Autodesk Inventor part; units mm, degrees
ref_plane "YZ Plane" through (0, 0, 0) normal (1, 0, 0) x (0, 1, 0)
ref_plane "XZ Plane" through (0, 0, 0) normal (0, 1, 0) x (-1, 0, 0)
ref_plane "XY Plane" through (0, 0, 0) normal (0, 0, 1) x (1, 0, 0)
sketch "Szkic1" plane through (0, 0, 0) normal (0, 1, 0) x (-1, 0, 0)
  line L0 (0, 0) -> (12.2, 0)
  line L1 (12.2, 0) -> (12.2, -22.6)
  line L2 (12.2, -22.6) -> (0, -22.6)
  line L3 (0, -22.6) -> (0, 0)
  dimension "d0" = 12.2
  dimension "d1" = 22.6
extrude "Wyciągnięcie proste1" add sketch "Szkic1" along normal blind 22.6
sketch "Szkic2" plane through (-12.2, 0, 0) normal (0, 0, 1) x (1, 0, 0)
  line L0 (0, 22.6) -> (12.2, 22.6) construction
  line L1 (0, 22.6) -> (0, 18.5) construction
  line L2 (0, 0) -> (0, 22.6) construction
  line L3 (0, 18.5) -> (12.2, 18.5) construction
  line L4 (12.2, 0) -> (12.2, 22.6) construction
  line L5 (0, 18.5) -> (0, 16.1) construction
  line L6 (0, 18.5) -> (12.2, 18.5)
  line L7 (12.2, 18.5) -> (12.2, 16.1)
  line L8 (12.2, 16.1) -> (0, 16.1)
  line L9 (0, 16.1) -> (0, 18.5)
  dimension "d4" = 4.1
  dimension "d5" = 2.4
extrude "Wyciągnięcie proste2" add sketch "Szkic2" along normal blind 4.5
sketch "Szkic3" plane through (0, 0, -22.6) normal (0, 0, -1) x (-1, 0, 0)
  line L0 (12.2, 18.5) -> (0, 18.5)
  line L1 (0, 16.1) -> (12.2, 16.1)
  line L2 (12.2, 0) -> (12.2, 22.6)
  line L3 (0, 0) -> (0, 22.6)
  line L4 (12.2, 18.5) -> (0, 18.5)
  line L5 (0, 18.5) -> (0, 16.1)
  line L6 (0, 16.1) -> (12.2, 16.1)
  line L7 (12.2, 16.1) -> (12.2, 18.5)
extrude "Wyciągnięcie proste3" add sketch "Szkic3" along normal blind 4.5
sketch "Szkic4" plane through (-12.2, 18.5, 0) normal (0, 1, 0) x (1, 0, 0)
  line L0 (0, -4.5) -> (12.2, -4.5) construction
  line L1 (6.1, -4.5) -> (6.1, 27) construction
  line L2 (6.1, -4.5) -> (5.6, -4.5) construction
  line L3 (6.1, -4.5) -> (6.1, -2.4) construction
  circle A0 centre (6.1, -2.4) radius 1 construction
  line L4 (5.6, -4.5) -> (6.6, -4.5) construction
  line L5 (6.6, -4.5) -> (6.6, -3) construction
  line L6 (6.6, -3) -> (5.6, -3) construction
  line L7 (5.6, -3) -> (5.6, -4.5) construction
  line L8 (5.6, -4.5) -> (5.6, -3.266)
  line L9 (5.6, -4.5) -> (6.6, -4.5)
  line L10 (6.6, -4.5) -> (6.6, -3.266)
  arc A1 (6.6, -3.266) -> (5.6, -3.266) centre (6.1, -2.4) ccw
  line L11 (0, 22.6) -> (0, 0) construction
  line L12 (0, 11.3) -> (12.2, 11.3) construction
  line L13 (12.2, 0) -> (12.2, 22.6) construction
  circle A2 centre (6.1, 25) radius 1 construction
  line L14 (5.6, 27.1) -> (6.6, 27.1) construction
  line L15 (5.6, 27.1) -> (5.6, 25.866)
  line L16 (6.6, 27.1) -> (6.6, 25.866)
  line L17 (5.6, 27.1) -> (6.6, 27.1)
  line L18 (0, 27.1) -> (12.2, 27.1)
  arc A3 (5.6, 25.866) -> (6.6, 25.866) centre (6.1, 25) ccw
  dimension "d10" = 0.5
  dimension "d11" = 2.1
  dimension "d12" = 2
  dimension "d13" = 1
extrude "Wyciągnięcie proste4" cut sketch "Szkic4" against normal blind 2.4
sketch "Szkic5" plane through (0, 22.6, 0) normal (0, 1, 0) x (1, 0, 0)
  line L0 (-12.2, 0) -> (0, 0) construction
  line L1 (-6.1, 0) -> (-6.1, 6.1) construction
  circle A0 centre (-6.1, 6.1) radius 6.1 construction
  line L2 (-6.1, 0) -> (-6.1, 14.5) construction
  circle A1 centre (-6.1, 12.2) radius 2.3 construction
  arc A2 (-8.3588, 11.7664) -> (-3.8412, 11.7664) centre (-6.1, 6.1) ccw
  arc A3 (-3.8412, 11.7664) -> (-8.3588, 11.7664) centre (-6.1, 12.2) ccw
  dimension "d16" = 6.1
  dimension "d17" = 12.2
  dimension "d18" = 14.5
extrude "Wyciągnięcie proste5" add sketch "Szkic5" along normal blind 4.1
sketch "Szkic6" plane through (0, 26.7, 0) normal (0, 1, 0) x (1, 0, 0)
  arc A0 (-8.3588, 11.7664) -> (-3.8412, 11.7664) centre (-6.1, 6.1) ccw
  circle A1 centre (-6.1, 6.1) radius 2.4
  point P0 (0, 0)
  dimension "d21" = 4.8
extrude "Wyciągnięcie proste6" add sketch "Szkic6" along normal blind 2.6
chamfer "Faza1" distance 2 angle 45 1 edges at (-6.1, 0, 0)
sketch "Szkic7" plane through (-12.2, 16.1, 0) normal (0, 0, 1) x (1, 0, 0)
  line L0 (12.2, -14.1) -> (0, -14.1) construction
  line L1 (6.1, -14.1) -> (6.1, -16.1) construction
  line L2 (0, -16.1) -> (12.2, -16.1) construction
  line L3 (6.1, -14.1) -> (4.35, -14.1) construction
  line L4 (4.35, -14.1) -> (7.85, -14.1)
  line L5 (7.85, -14.1) -> (7.85, -15.5)
  line L6 (7.85, -15.5) -> (4.35, -15.5)
  line L7 (4.35, -15.5) -> (4.35, -14.1)
  dimension "d27" = 1.75
  dimension "d28" = 3.5
  dimension "d29" = 1.4
extrude "Wyciągnięcie proste7" add sketch "Szkic7" along normal blind 1 and the other way blind 1.3
properties part number "SG92r"
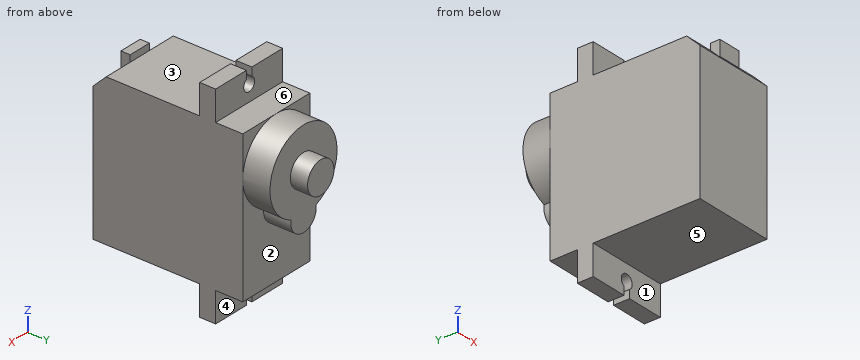
For this review, take the finished solid that the model builds, in its own axes (mm). Face numbers are marked on the shaded views. A direction names the side the tool comes from. Round coordinates to 2 decimals unless told otherwise and drop trailing zeros. Write each loop counter-clockwise with the first axis right and the second up, starting at its lowest first coordinate (ties: lowest second). Pieces come first, ordered by that corner, then holes. Notation, with made-up numbers: (-36, 84.25) - (21, 84.25) arc R21 ccw to (21, 89.25) - close; hole circle Ø9 at (53.25, -28.75). An arc over 180 degrees is marked (long way). Use a Markdown table: item, result.
Q1. Wall thickness on line 1 along X through (y, z) = (17.6, 2.4); line 2 along Z through (x, y) = (-7, 17.5); line 3 along Y through (x, z) = (-8.25, -23.5): over which ranges is each line inside the solid? List them lowest first.
Derived:
| item | result |
|---|---|
| line 1 | x = -12.2 to -7.1, -5.1 to 0 |
| line 2 | z = -27.1 to -25.44, -24.56 to 1.96, 2.84 to 4.5 |
| line 3 | y = 16.1 to 18.5 |
Q2. Clearance check with flat-ended pins moving along their axes: pin 1 (1.3 mm diameter, centred on x = -6.5, z = 3, fed in from +Y); pin 2 (3 mm diameter, centred on x = -6, y = 24, fed in from -Z); pin 3 (1.5 mm diameter, centred on x = -5.5, z = -13, fed in from +Y). State where each tip first meets the part, or that it passes through.
Derived:
| item | result |
|---|---|
| pin 1 | stops at y = 18.5 |
| pin 2 | stops at z = -22.6 |
| pin 3 | stops at y = 26.7 |
Q3. The part is to be moulded in two halves that separate along Y. For the marked faces 1, 2 and 3, say which applies: pulls with the +Y half, pulls with the -Y half, needs draft (parallel to the pull), parting line crosses it, or undercut.
Derived:
| item | result |
|---|---|
| face 1 | pulls with the -Y half |
| face 2 | pulls with the +Y half |
| face 3 | undercut |
Q4. We need section B-B (x = -10.5). Give the boundary of the cut face in (y, z).
Derived:
| item | result |
|---|---|
| outline | (0, -22.6) - (16.1, -22.6) - (16.1, -27.1) - (18.5, -27.1) - (18.5, -22.6) - (22.6, -22.6) - (22.6, -10.32) - (26.7, -10.32) - (26.7, -1.88) - (22.6, -1.88) - (22.6, 0) - (18.5, 0) - (18.5, 4.5) - (16.1, 4.5) - (16.1, 0) - (2, 0) - (0, -2) - close |
Q5. We need section A-A (z = -25). Give the boundary of the cut face in (x, y), plus the area to 3 significant figures.
Derived:
| item | result |
|---|---|
| outline | (-12.2, 16.1) - (-7.1, 16.1) - (-7.1, 18.5) - (-12.2, 18.5) - close; (-5.1, 16.1) - (0, 16.1) - (0, 18.5) - (-5.1, 18.5) - close |
| area | 24.5 mm2 |
Q6. We need section C-C (z = -12.2). Give the boundary of the cut face in (x, y).
Derived:
| item | result |
|---|---|
| outline | (-12.2, 0) - (0, 0) - (0, 22.6) - (-3.8, 22.6) - (-3.8, 26.7) - (-8.4, 26.7) - (-8.4, 22.6) - (-12.2, 22.6) - close |
Q7. Machinability: for the marked faces 4, 5 and 6, which of the approach directions +Z, -Z, +X, -X, +Y, -Y give a long, thin tool a straight path to every point of the face, cutting with its end or side? Answer none if there is none.
Derived:
| item | result |
|---|---|
| face 4 | -Z, +X, -X, +Y |
| face 5 | -Z, +X, -X, -Y |
| face 6 | +Z, +X, -X, +Y |
Q8. We need section D-D (y = 19.25). Give the boundary of the cut face in (x, z), plus the area to 3 significant figures.
Derived:
| item | result |
|---|---|
| outline | (-12.2, -22.6) - (0, -22.6) - (0, 0) - (-12.2, 0) - close |
| area | 276 mm2 |
